Verification items for the finished model (mm, model axes). Give positions to 0.01 mm unless a question says otherwise; leave off trailing zeros. Order: outer loops, then holes, each group sorted by start corner. A loop starts at its lowest first (then second) coordinate and runs counter-clockwise, first axis right, second up. Notation, with made-up numbers: (9.5, 56) -> (56.5, 56) arc R19 ccw to (56.5, 81) -> close; hole circle Ø10 at (49.5, -6). An arc over 180 degrees is marked (long way). Return JSON: item names as keys, results as strings. Group by question number.
(1) Cross-section at C-C on y = 46. Enter the section's corners in (x, z).
(2) Cross-section at A-A on z = -100. Enter the section's corners in (x, y), then the cut area to 3 significant figures.
(3) Cross-section at B-B on z = -150.5. Enter the section's corners in (x, y), then the cut area to 3 significant figures.
(4) Depth check by flat-ended pin: pin 1 Ø1.5 at (x, y) = (87.5, 1.5) entering from -Z; pin 2 Ø1.5 at (x, y) = (-87, 1.5) entering from +Z; pin 3 Ø8 at (y, z) = (54, 50.5) entering from +X. Enter the tip coordinate at first touch or a pass-through.
(5) Thickness scan on line 1 along X through (y, z) = (14, 46); line 2 along X through (y, z) = (66, 136.5). Record the ranges inside material, lowest first.
from build123d import *

# Parameters (mm, degrees)
CROQUIS1_W              = 160
CROQUIS1_H              = 70
SALIENTE_EXTRUIR1_DEPTH = 173
CROQUIS2_W              = 12
CROQUIS2_H              = 343
SALIENTE_EXTRUIR2_DEPTH = 3
CORTAR_EXTRUIR1_DEPTH   = 4
REDONDEO1_R             = 5


with BuildPart() as part:
    # Croquis1 → Saliente-Extruir1 (new body, symmetric)
    with BuildSketch(Plane.XY):
        with Locations((0, 35)):
            Rectangle(CROQUIS1_W, CROQUIS1_H)
    extrude(amount=SALIENTE_EXTRUIR1_DEPTH, both=True)

    # Croquis2 → Saliente-Extruir2 (add)
    with BuildSketch(Plane.XZ):
        with Locations((86, 0)):
            Rectangle(CROQUIS2_W, CROQUIS2_H)
    extrude(amount=-SALIENTE_EXTRUIR2_DEPTH)

    # Croquis3 → Cortar-Extruir1 (cut, through all)
    with BuildSketch(Plane(origin=(0, 3, 0), x_dir=(1, 0, 0), z_dir=(0, 1, 0))):
        with BuildLine():
            Line((85, -103.5), (92, -103.5))
            Line((92, -103.5), (92, -96.5))
            Line((92, -96.5), (85, -96.5))
            ThreePointArc((85, -96.5), (81.5, -100), (85, -103.5))
        make_face()
    cortar_extruir1 = extrude(amount=-CORTAR_EXTRUIR1_DEPTH, mode=Mode.SUBTRACT)

    # Simetría1: Cortar-Extruir1 across plane
    add(cortar_extruir1.mirror(Plane.XY), mode=Mode.SUBTRACT)

    # Simetría5: part across plane


with BuildPart() as part_1:
    add(part.part)
    add(part.part.mirror(Plane(origin=(0, 0, 0), x_dir=(0, 0, 1), z_dir=(1, 0, 0))))

    # Redondeo1
    redondeo1_edges = [part_1.edges().sort_by_distance(p)[0] for p in [
        (92, 1.5, 171.5),
        (92, 1.5, -171.5),
        (-92, 1.5, -171.5),
        (-92, 1.5, 171.5),
        (-80, 70, 0),
        (80, 70, 0),
    ]]
    fillet(redondeo1_edges, radius=REDONDEO1_R)


solid = part_1.part
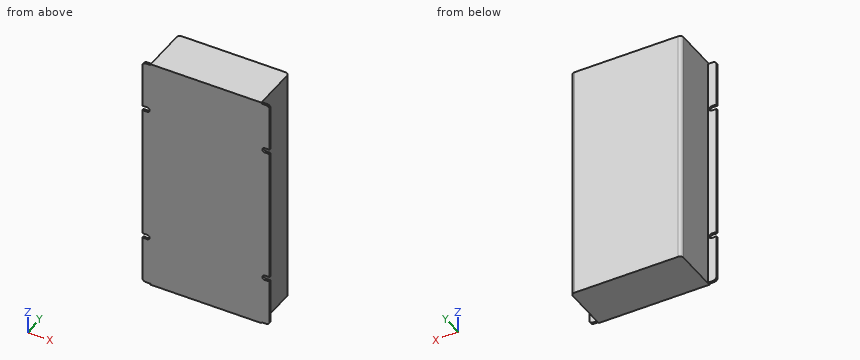
Verdict:
{
 "1": {"outline": "(-80, -173) -> (80, -173) -> (80, 173) -> (-80, 173) -> close"},
 "2": {"outline": "(-81.5, 0) -> (81.5, 0) -> (81.5, 3) -> (80, 3) -> (80, 65) arc R5 ccw to (75, 70) -> (-75, 70) arc R5 ccw to (-80, 65) -> (-80, 3) -> (-81.5, 3) -> close", "area": "11,200 mm²"},
 "3": {"outline": "(-92, 0) -> (92, 0) -> (92, 3) -> (80, 3) -> (80, 65) arc R5 ccw to (75, 70) -> (-75, 70) arc R5 ccw to (-80, 65) -> (-80, 3) -> (-92, 3) -> close", "area": "11,300 mm²"},
 "4": {"pin 1": "z = -171.5", "pin 2": "z = 171.5", "pin 3": "x = 80"},
 "5": {"line 1": "-80 to 80", "line 2": "-79.9 to 79.9"}
}
